Can you work these out from the model? Positions are in its coordinate system, mm. A direction names the side the tool comes from. Round coordinates to 2 decimals unless told otherwise and drop trailing zeros. Write each loop counter-clockwise with the first axis right and the second up, starting at its lowest first coordinate (ties: lowest second). Pieces come first, ordered by that corner, then holes. Notation, with made-up numbers: M -37,-8 L -4,-8 A14 ccw -4,7 Z; hole C 0,65 d10. An arc over 180 degrees is marked long. Answer in a Markdown table with one row per item. Add a question column.
(1) Suppose I cut it at A-A, the plane x = 15. Write out the boundary of the cut face in (y, z), then the cut area to 3 significant figures.
(2) Suppose I cut it at C-C, the plane y = 12. Write out the boundary of the cut face in (x, z).
(3) I'm going to push flat-ended pins straight in: pin 1 (9.5 mm diameter, centred on y = 28.5, z = 15, fed in from -X); pin 2 (6 mm diameter, centred on x = 19, y = 6.5, fed in from +Z); pin 3 (3.5 mm diameter, centred on y = 27.5, z = 18, fed in from +X). Where does each tip first touch, or does it pass through?
(4) For faces 1 (the face through (10, 20, 15)), 2 (the face through (15, 0, 15)), 3 (the face through (15, 20, 10)), 4 (the face through (15, 18, 20)), which set-ups out of +Z, -Z, +X, -X, +Y, -Y let a thin tool reach every point of the face, with its end or its side?
(5) Suppose I cut it at B-B, the plane z = 19.25. Write out the boundary of the cut face in (x, y).
(6) If we mould it in two halves opening along Y, with no side actions, what happens to faces 5 (the face through (20, 20, 15)), 6 (the face through (14.93, 35.12, 20.83)), 7 (the face through (14.93, 39.787, 10.833))? For each: released by +Y, released by -Y, zero draft, split by the parting line, or undercut.
(7) Suppose I cut it at D-D, the plane z = 27.5. Write out the boundary of the cut face in (x, y).
(8) If I drill on probe 1 along Y at (x, z) = (9.25, 22.25); probe 2 along X at (y, z) = (26, 14.5), over which ranges is the centre line in solid material (lowest first)?
from build123d import *

# Parameters (mm, degrees)
SKETCH1_W           = 30
SKETCH1_H           = 30
BOSS_EXTRUDE1_DEPTH = 3
SKETCH2_W           = 10
SKETCH2_H           = 10
BOSS_EXTRUDE2_DEPTH = 35
CUT_EXTRUDE2_DEPTH  = 21
SKETCH5_W           = 10
SKETCH5_H           = 11.03377919
BOSS_EXTRUDE3_DEPTH = 4


with BuildPart() as part:
    # Sketch1 → Boss-Extrude1 (new body)
    with BuildSketch(Plane(origin=(0, 0, 0), x_dir=(1, 0, 0), z_dir=(0, 1, 0))):
        with Locations((15, -15)):
            Rectangle(SKETCH1_W, SKETCH1_H)
    extrude(amount=BOSS_EXTRUDE1_DEPTH)

    # Sketch2 → Boss-Extrude2 (add)
    with BuildSketch(Plane(origin=(0, 3, 0), x_dir=(1, 0, 0), z_dir=(0, 1, 0))):
        with Locations((15, -15)):
            Rectangle(SKETCH2_W, SKETCH2_H)
    extrude(amount=BOSS_EXTRUDE2_DEPTH)

    # Sketch3 → Cut-Extrude2 (cut, through all)
    with BuildSketch(Plane(origin=(20, 0, 0), x_dir=(0, 0, -1), z_dir=(1, 0, 0))):
        Polygon((-20, 38), (-10, 38), (-20, 33.336923418), align=None)
    extrude(amount=-CUT_EXTRUDE2_DEPTH, mode=Mode.SUBTRACT)

    # Sketch5 → Boss-Extrude3 (add)
    with BuildSketch(Plane(origin=(0, 35.0431868, 16.340906371), x_dir=(1, 0, 0), z_dir=(0, 0.906307787, 0.422618262))):
        with Locations((15, 1.479526481)):
            Rectangle(SKETCH5_W, SKETCH5_H)
    extrude(amount=BOSS_EXTRUDE3_DEPTH)


solid = part.part
Calculated:
| question | item | result |
|---|---|---|
| 1 | outline | M 0,0 L 3,0 L 3,10 L 38,10 L 41.63,11.69 L 36.96,21.69 L 33.34,20 L 3,20 L 3,30 L 0,30 Z |
| 1 | area | 461 mm² |
| 2 | outline | M 10,10 L 20,10 L 20,20 L 10,20 Z |
| 3 | pin 1 | x = 10 |
| 3 | pin 2 | z = 20 |
| 3 | pin 3 | x = 20 |
| 4 | face 1 | +Z, -Z, -X, +Y |
| 4 | face 2 | +Z, -Z, +X, -X, -Y |
| 4 | face 3 | -Z, +X, -X, +Y |
| 4 | face 4 | +Z, +X, -X |
| 5 | outline | M 0,0 L 30,0 L 30,3 L 20,3 L 20,38.1 L 10,38.1 L 10,3 L 0,3 Z |
| 6 | face 5 | zero draft |
| 6 | face 6 | undercut |
| 6 | face 7 | released by +Y |
| 7 | outline | M 0,0 L 30,0 L 30,3 L 0,3 Z |
| 8 | probe 1 | 0 to 3 |
| 8 | probe 2 | 10 to 20 |
